Source: three-view drawing plus pictorial views. Frame: mm from the lowest corner of the part. A direction names the side the tool comes from. Coordinates: 2 decimals unless noted, no trailing zeros. Write each loop counter-clockwise with the first axis right and the second up, starting at its lowest first coordinate (ties: lowest second). Pieces come first, ordered by that corner, then holes. Notation, with made-up numbers: (75.25, 51.25) -> (109.25, 51.25) arc R11 ccw to (109.25, 61.25) -> close; hole circle Ø2 at (45, -11.5). An arc over 180 degrees is marked (long way). One line per item, written item: value.
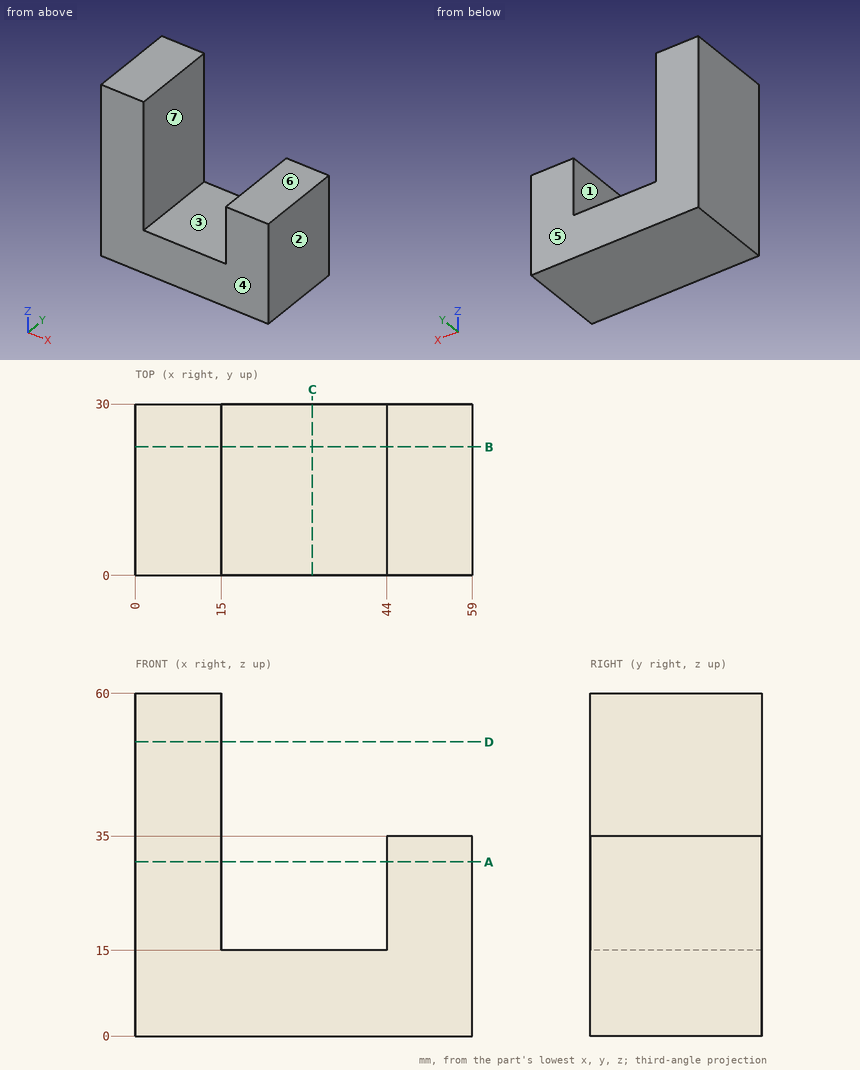
(1) Pull-direction query (X, two-part tool) for the marked faces 1, 2, 3 and 4; classes: released by +X, released by -X, zero draft, split by the parting line, or undercut.
Responses:
face 1: undercut
face 2: released by +X
face 3: undercut
face 4: zero draft
(2) Section B-B (y = 22.5). Return the cut outline in (x, z).
Responses:
outline: (0, 0) -> (59, 0) -> (59, 35) -> (44, 35) -> (44, 15) -> (15, 15) -> (15, 60) -> (0, 60) -> close
(3) Section C-C (x = 31). Return the cut outline in (y, z).
Responses:
outline: (0, 0) -> (30, 0) -> (30, 15) -> (0, 15) -> close
(4) First-contact query: pin 1 (6 mm diameter, centred on x = 24, y = 14.5, fed in from +Z); pin 2 (12 mm diameter, centred on x = 51.5, y = 19, fed in from +Z). Flat tips, straight axial feed; report the tip coordinate or a pass-through.
Responses:
pin 1: stops at z = 15
pin 2: stops at z = 35
(5) Line query: line 1 (X direction, y = 4, z = 29); line 2 (Z direction, x = 17.5, y = 23); line 3 (Z direction, x = 50.5, y = 17). Output: solid intervals per line, ascending. Write a range as [from, to].
Responses:
line 1: x = [0, 15], [44, 59]
line 2: z = [0, 15]
line 3: z = [0, 35]
(6) Section D-D (z = 51.5). Return the cut outline in (x, y), then the cut area to 3 significant figures.
Responses:
outline: (0, 0) -> (15, 0) -> (15, 30) -> (0, 30) -> close
area: 450 mm2
(7) Reachability of the marked faces 5, 6 and 7 from +Z, -Z, +X, -X, +Y, -Y: full face, straight path, thin tool, end or side. Return the list, or none.
Responses:
face 5: +Z, -Z, +X, -X, +Y
face 6: +Z, +X, +Y, -Y
face 7: +Z, +Y, -Y
(8) Section A-A (z = 30.5). Return the cut outline in (x, y).
Responses:
outline: (0, 0) -> (15, 0) -> (15, 30) -> (0, 30) -> close; (44, 0) -> (59, 0) -> (59, 30) -> (44, 30) -> close
